Can you work these out from the model? Positions are in its coordinate system, mm. Give positions to 0.01 mm unless a question says otherwise; leave off trailing zeros. Loops run counter-clockwise (first coordinate to the right, second up) from the corner with the lowest first, then second, coordinate; pieces in that order, holes last. Notation, with made-up numbers: (-9, 38) -> (-4, 38) arc R21 ccw to (-4, 63) -> close; hole circle Ø11 at (79.5, 10). An arc over 180 degrees is marked (long way). Return JSON: item names as keys, results as strings. Group by question number.
Q1. I need wall thicknesses on line 1 along Z through (x, y) = (747, -9); line 2 along Z through (x, y) = (475.5, 6.25); line 3 along X through (y, z) = (-11, -1.5). Which ranges of each line are inside material? Lowest first, please. Write a range as [from, to].
Q2. Will these pins go through, and if not, where does the flat tip stop? pin 1 (4 mm diameter, centred on x = 591.5, z = -5.5, fed in from -Y); pin 2 (10 mm diameter, centred on x = 306.5, y = -0.5, fed in from +Z); pin 3 (8 mm diameter, centred on x = 365.5, z = 5.5, fed in from +Y); pin 4 (2 mm diameter, centred on x = 850, z = -6.5, fed in from +Y).
Q3. Suppose I cut it at A-A, the plane x = 141. Please give me the cut outline in (y, z).
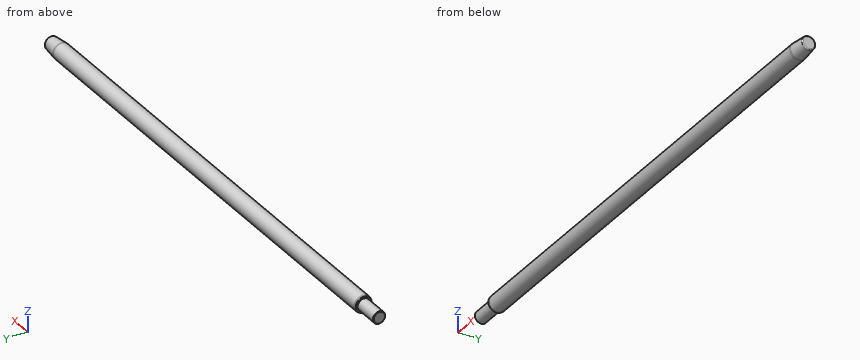
```python
from build123d import *

# Parameters (mm, degrees)
F0_R     = 11
F1_DEPTH = 45
F2_R     = 15
F2_R_2   = 11
F3_DEPTH = 900
F4_SIZE2 = 3.153127058
F4_SIZE  = 30
F5_SIZE  = 1
F6_SIZE2 = 0.8038475773
F6_SIZE  = 3
F7_R     = 0.5
F8_R     = 5
F9_R     = 20
F10_R    = 2


with BuildPart() as f1:
    # F0 (on Right) → F1 (new body)
    with BuildSketch(Plane.YZ):
        Circle(F0_R)
    extrude(amount=F1_DEPTH)

    # F2 (on face) → F3 (join)
    with BuildSketch(Plane.YZ.offset(45)):
        Circle(F2_R)
        Circle(F2_R_2, mode=Mode.SUBTRACT)
        Circle(F2_R_2)
    extrude(amount=F3_DEPTH)

    # F4
    f4_edges = [f1.edges().sort_by_distance(p)[0] for p in [
        (945, -15, 0),
    ]]
    f4_side = f1.faces().sort_by_distance((495, -15, 0))[0]
    chamfer(f4_edges, length=F4_SIZE, length2=F4_SIZE2, reference=f4_side)

    # F5
    f5_edges = [f1.edges().sort_by_distance(p)[0] for p in [
        (0, -11, 0),
    ]]
    chamfer(f5_edges, length=F5_SIZE)

    # F6
    f6_edges = [f1.edges().sort_by_distance(p)[0] for p in [
        (45, -15, 0),
    ]]
    f6_side = f1.faces().sort_by_distance((480, -15, 0))[0]
    chamfer(f6_edges, length=F6_SIZE, length2=F6_SIZE2, reference=f6_side)

    # F7
    f7_edges = [f1.edges().sort_by_distance(p)[0] for p in [
        (45, -11, 0),
        (45, -14.196152, 0),
    ]]
    fillet(f7_edges, radius=F7_R)

    # F8
    f8_edges = [f1.edges().sort_by_distance(p)[0] for p in [
        (48, -15, 0),
    ]]
    fillet(f8_edges, radius=F8_R)

    # F9
    f9_edges = [f1.edges().sort_by_distance(p)[0] for p in [
        (915, -15, 0),
    ]]
    fillet(f9_edges, radius=F9_R)

    # F10
    f10_edges = [f1.edges().sort_by_distance(p)[0] for p in [
        (945, -11.846873, 0),
    ]]
    fillet(f10_edges, radius=F10_R)


solid = f1.part
```
Ans:
{
 "1": {"line 1": "z = [-12, 12]", "line 2": "z = [-13.64, 13.64]", "line 3": "x = [44.8, 944.7]"},
 "2": {"pin 1": "stops at y = -14.59", "pin 2": "stops at z = 15", "pin 3": "stops at y = 14.92", "pin 4": "stops at y = 13.96"},
 "3": {"outline": "circle Ø30 at (0, 0)"}
}
